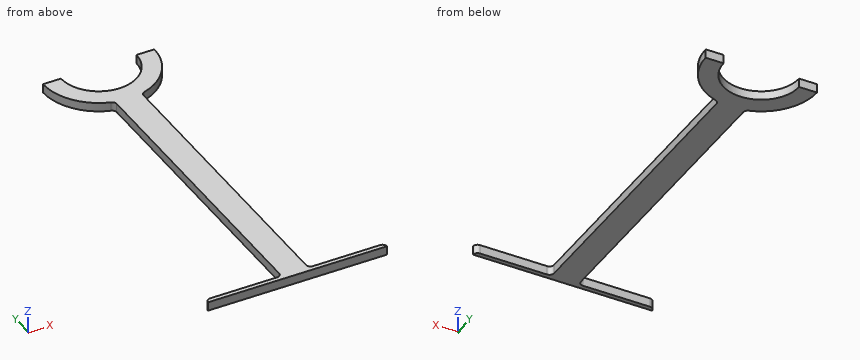
from build123d import *

# Parameters (mm, degrees)
BOSS_EXTRUDE1_DEPTH      = 2.5
SKETCH3_W                = 15
SKETCH3_H                = 175
BOSS_EXTRUDE2_DEPTH      = 2.5
BOSS_EXTRUDE4_DEPTH      = 50
BOSS_EXTRUDE4_DEPTH_BACK = 50
SKETCH5_W                = 5
SKETCH5_H                = 2.5
FILLET1_R                = 2.5
FILLET2_R                = 2.5
FILLET3_R                = 2.5
FILLET4_R                = 2.5
FILLET5_R                = 2.5
FILLET6_R                = 2.5


with BuildPart() as part:
    # Sketch1 → Boss-Extrude1 (new, symmetric)
    with BuildSketch(Plane.XY):
        with BuildLine():
            Line((-21.1, 0), (-31.1, 0))
            ThreePointArc((-31.1, 0), (0, -31.1), (31.1, 0))
            Line((31.1, 0), (21.1, 0))
            ThreePointArc((21.1, 0), (0, -21.1), (-21.1, 0))
        make_face()
    extrude(amount=BOSS_EXTRUDE1_DEPTH, both=True)

    # Sketch3 → Boss-Extrude2 (add, symmetric)
    with BuildSketch(Plane.XY):
        with Locations((0, -115.239187588)):
            Rectangle(SKETCH3_W, SKETCH3_H)
    extrude(amount=BOSS_EXTRUDE2_DEPTH, both=True)

    # Sketch5 → Boss-Extrude4 (add, two sides: drawn at the far end of the back side and taken through both)
    with BuildSketch(Plane(origin=(0, 0, 0), x_dir=(0, 0, -1), z_dir=(1, 0, 0)).offset(-BOSS_EXTRUDE4_DEPTH_BACK)):
        with Locations((0, -201.489187588)):
            Rectangle(SKETCH5_W, SKETCH5_H)
    extrude(amount=BOSS_EXTRUDE4_DEPTH + BOSS_EXTRUDE4_DEPTH_BACK)

    # Fillet1
    fillet1_edges = [part.edges().sort_by_distance(p)[0] for p in [
        (7.5, -200.239187588, 0),
    ]]
    fillet(fillet1_edges, radius=FILLET1_R)

    # Fillet2
    fillet2_edges = [part.edges().sort_by_distance(p)[0] for p in [
        (-7.5, -200.239187588, 0),
    ]]
    fillet(fillet2_edges, radius=FILLET2_R)

    # Fillet3
    fillet3_edges = [part.edges().sort_by_distance(p)[0] for p in [
        (7.5, -30.182113909, 0),
    ]]
    fillet(fillet3_edges, radius=FILLET3_R)

    # Fillet4
    fillet4_edges = [part.edges().sort_by_distance(p)[0] for p in [
        (-7.5, -30.182113909, 0),
    ]]
    fillet(fillet4_edges, radius=FILLET4_R)

    # Fillet5
    fillet5_edges = [part.edges().sort_by_distance(p)[0] for p in [
        (50, -200.239187588, 0),
    ]]
    fillet(fillet5_edges, radius=FILLET5_R - 0.0001)  # a hair under: the kernel refuses the full size

    # Fillet6
    fillet6_edges = [part.edges().sort_by_distance(p)[0] for p in [
        (-50, -200.239187588, 0),
    ]]
    fillet(fillet6_edges, radius=FILLET6_R - 0.0001)  # a hair under: the kernel refuses the full size


solid = part.part
Design review of the part built by this model. Coordinates are the model's own, in mm. Round coordinates to 2 decimals unless told otherwise and drop trailing zeros. Write each loop counter-clockwise with the first axis right and the second up, starting at its lowest first coordinate (ties: lowest second). Pieces come first, ordered by that corner, then holes. Notation, with made-up numbers: (-29.5, 0) -> (19.5, 0) arc R23 ccw to (19.5, 28) -> close; hole circle Ø6 at (10, 68). An arc over 180 degrees is marked (long way). One line per item, written item: value. Start each with the question number.
Q1. Insertion check: P1, Ø2.5, axis at y = -110.5, z = 0.5, coming from the +X side; P2, Ø2.5, axis at x = 34, z = -1, coming from the +Y side; P3, Ø1, axis at y = -46.5, z = -1.5, coming from the -X side. Each pin has a flat end and moves straight along its axis. Give the tip position at first contact, or say it passes through.
Q2. Add section C-C (y = -44). Give the boundary of the cut face in (x, z).
Q3. Add section B-B (x = 0). Give the boundary of the cut face in (y, z).
Q4. To check wall thickness, follow probe 1 along Y at (x, z) = (-36, -1.8); probe 2 along X at (y, z) = (-89.5, 0.75); probe 3 along Y at (x, z) = (-25.5, 1.8). State the ranges of each line that lie inside material, in increasing order.
Response:
1. P1: stops at x = 7.5
1. P2: stops at y = -200.24
1. P3: stops at x = -7.5
2. outline: (-7.5, -2.5) -> (7.5, -2.5) -> (7.5, 2.5) -> (-7.5, 2.5) -> close
3. outline: (-202.74, -2.5) -> (-21.1, -2.5) -> (-21.1, 2.5) -> (-202.74, 2.5) -> close
4. probe 1: y = -202.74 to -200.24
4. probe 2: x = -7.5 to 7.5
4. probe 3: y = -202.74 to -200.24, -17.8 to 0
